Input: dimensioned drawing with shaded views. Units: mm. Origin: part minimum x, y, z. A direction names the side the tool comes from. Coordinates: 2 decimals unless noted, no trailing zeros. Loops run counter-clockwise (first coordinate to the right, second up) from the corner with the lowest first, then second, coordinate; pieces in that order, holes last. Notation, with made-up numbers: (-14.5, -36.75) -> (8.5, -36.75) arc R25 cw to (8.5, -6.75) -> close; hole circle Ø4 at (-12, -36.75). An arc over 180 degrees is marked (long way). Answer as CSV lines item,"result".
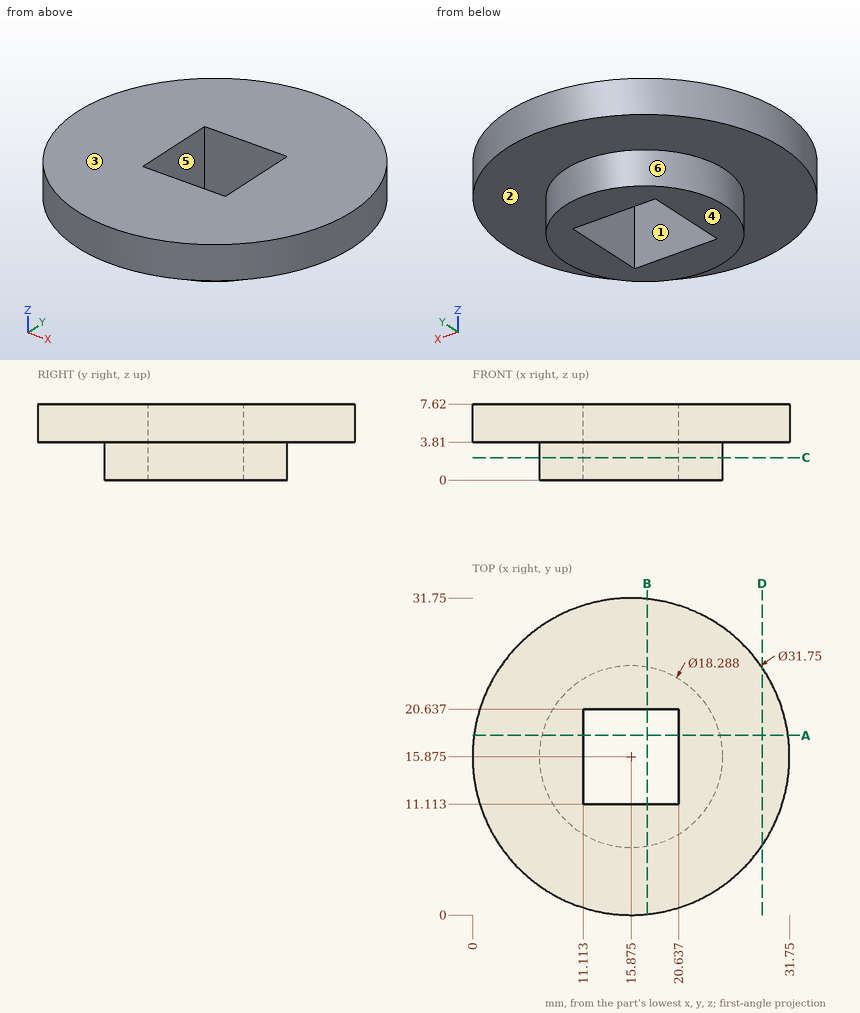
(1) Pin query (flat end, axial travel): pin 1 Ø1 at (y, z) = (11, 1.5) entering from -X (1 decimal); pin 2 Ø1 at (y, z) = (8.5, 3) entering from -X (1 decimal); pin 3 Ø3 at (y, z) = (19.5, 3.5) entering from +X. Return the tip coordinate at first contact, or that it passes through.
Computed values:
pin 1,"x = 7.8"
pin 2,"x = 9.8"
pin 3,"x = 31.6"
(2) Cut plane B-B (x = 17.5). Return the cut outline in (y, z), then the cut area to 3 significant figures.
Computed values:
outline,"(0.08, 3.81) -> (6.88, 3.81) -> (6.88, 0) -> (11.11, 0) -> (11.11, 7.62) -> (0.08, 7.62) -> close; (20.64, 0) -> (24.87, 0) -> (24.87, 3.81) -> (31.67, 3.81) -> (31.67, 7.62) -> (20.64, 7.62) -> close"
area,"116 mm^2"
(3) Access query for the marked faces 1, 2 and 3. Directions: +Z, -Z, +X, -X, +Y, -Y. A direction counts if a zero-diameter tool reaches every point of the face in a straight line with its end or side. Return the directions, or none.
Computed values:
face 1,"+Z, -Z"
face 2,"-Z"
face 3,"+Z, +X, -X, +Y, -Y"
(4) Material intervals for L1, parallel to Y at x = 15.5, z = 4 (1 decimal); L2, parallel to Z at x = 29, y = 15; L3, parallel to Y at x = 18.5, z = 6.5, sorted ascending. Write a range as [from, to].
Computed values:
L1,"[0, 11.1], [20.6, 31.7]"
L2,"[3.81, 7.62]"
L3,"[0.22, 11.11], [20.64, 31.53]"
(5) Cut plane D-D (x = 29). Return the cut outline in (y, z) (1 decimal).
Computed values:
outline,"(6.9, 3.8) -> (24.8, 3.8) -> (24.8, 7.6) -> (6.9, 7.6) -> close"
(6) Draft query along X for the marked faces 4, 5 and 6. Return one class per face: released by +X, released by -X, zero draft, split by the parting line, or undercut.
Computed values:
face 4,"zero draft"
face 5,"undercut"
face 6,"split by the parting line"
(7) Cut plane C-C (z = 2.25). Return the cut outline in (x, y) (1 decimal).
Computed values:
outline,"circle Ø18.3 at (15.9, 15.9); hole (11.1, 11.1) -> (20.6, 11.1) -> (20.6, 20.6) -> (11.1, 20.6) -> close"
(8) Cut plane A-A (y = 18). Return the cut outline in (x, z).
Computed values:
outline,"(0.14, 3.81) -> (6.98, 3.81) -> (6.98, 0) -> (11.11, 0) -> (11.11, 7.62) -> (0.14, 7.62) -> close; (20.64, 0) -> (24.77, 0) -> (24.77, 3.81) -> (31.61, 3.81) -> (31.61, 7.62) -> (20.64, 7.62) -> close"
